```python
from build123d import *

# Parameters (mm, degrees)
BOSS_EXTRUDE1_DEPTH                            = 4
SKETCH3_R                                      = 2.15
BOSS_EXTRUDE2_DEPTH                            = 8
BOSS_EXTRUDE3_DEPTH                            = 8
CUT_EXTRUDE2_REACH                             = 34.144
SKETCH4_R                                      = 2.25
SKETCH4_4_W                                    = 12.7
SKETCH4_4_H                                    = 12.7
SKETCH4_4_R                                    = 2.25
CUT_EXTRUDE3_DEPTH                             = 8.5
BOSS_EXTRUDE4_DEPTH                            = 5.8
BOSS_EXTRUDE7_DEPTH                            = 3
CBORE_FOR_6_SOCKET_HEAD_CAP_SCREW1_D           = 3.6576
CBORE_FOR_6_SOCKET_HEAD_CAP_SCREW1_CBORE_D     = 7.14502
CBORE_FOR_6_SOCKET_HEAD_CAP_SCREW1_CBORE_DEPTH = 3.5052
SKETCH12_R                                     = 1.75
BOSS_EXTRUDE8_DEPTH                            = 2
CHAMFER1_SIZE                                  = 5
FILLET1_R                                      = 1


with BuildPart() as part:
    # Sketch2 → Boss-Extrude1 (new body)
    with BuildSketch(Plane.XY):
        with BuildLine():
            Line((15.5, 0), (20, 4.5))
            Line((20, 4.5), (20, 27))
            Line((20, 27), (1, 27))
            ThreePointArc((1, 27), (0.292893219, 26.707106781), (0, 26))
            Line((0, 26), (0, 1))
            ThreePointArc((0, 1), (0.292893219, 0.292893219), (1, 0))
            Line((1, 0), (15.5, 0))
        make_face()
    extrude(amount=BOSS_EXTRUDE1_DEPTH)

    # Sketch3 → Boss-Extrude2 (add)
    with BuildSketch(Plane.XY):
        with Locations((4.5, 22.5)):
            Circle(SKETCH3_R)
        with Locations((4.5, 4.5)):
            Circle(SKETCH3_R)
    extrude(amount=-BOSS_EXTRUDE2_DEPTH)

    # Sketch3<3> → Boss-Extrude3 (add)
    with BuildSketch(Plane.XY):
        with BuildLine():
            Line((4.5, 15), (4.5, 12))
            ThreePointArc((4.5, 12), (8.782801805, 10.656915518), (11.531693039, 7.108695652))
            ThreePointArc((11.531693039, 7.108695652), (12.997768364, 5.216311724), (15.281929326, 4.5))
            Line((15.281929326, 4.5), (20, 4.5))
            Line((20, 4.5), (20, 27))
            Line((20, 27), (12, 27))
            Line((12, 27), (12, 22.5))
            ThreePointArc((12, 22.5), (9.803300859, 17.196699141), (4.5, 15))
        make_face()
    extrude(amount=-BOSS_EXTRUDE3_DEPTH)

    # Cut-Extrude2: up to this face of the body (flat: up to its plane)
    cut_extrude2_end = Plane(part.part.faces().sort_by_distance((20, 15.75, -2))[0])
    # Sketch4 → Cut-Extrude2 (cut, up to the picked face)
    with BuildSketch(Plane(origin=(4.5, 0, 0), x_dir=(0, 0, -1), z_dir=(1, 0, 0)), mode=Mode.PRIVATE) as cut_extrude2_sk1:
        with Locations((8, 13.5)):
            Circle(SKETCH4_R)
    cut_extrude2_tool1 = split(extrude(cut_extrude2_sk1.sketch, amount=CUT_EXTRUDE2_REACH, mode=Mode.PRIVATE), bisect_by=cut_extrude2_end, keep=Keep.BOTH, mode=Mode.PRIVATE)
    add(cut_extrude2_tool1.solids().sort_by(Axis((4.5, 13.5, -8), (1, 0, 0)))[0], mode=Mode.SUBTRACT)

    # Sketch4<4> → Cut-Extrude3 (cut)
    with BuildSketch(Plane(origin=(4.5, 0, 0), x_dir=(0, 0, -1), z_dir=(1, 0, 0))):
        with Locations((8, 13.5)):
            Rectangle(SKETCH4_4_W, SKETCH4_4_H)
        with Locations((8, 13.5)):
            Circle(SKETCH4_4_R, mode=Mode.SUBTRACT)
    extrude(amount=CUT_EXTRUDE3_DEPTH, mode=Mode.SUBTRACT)

    # Sketch5 → Boss-Extrude4 (add)
    with BuildSketch(Plane(origin=(20, 0, 0), x_dir=(0, 0, -1), z_dir=(1, 0, 0))):
        with BuildLine():
            Line((1.45, 4.5), (1.45, 9.745003329))
            ThreePointArc((1.45, 9.745003329), (1.467285217, 17.28498845), (8, 21.05))
            Line((8, 21.05), (8, 27))
            Line((8, 27), (-4, 27))
            Line((-4, 27), (-4, 4.5))
            Line((-4, 4.5), (0, 4.5))
            Line((0, 4.5), (1.45, 4.5))
        make_face()
    extrude(amount=BOSS_EXTRUDE4_DEPTH)

    # Sketch8 → Boss-Extrude7 (add)
    with BuildSketch(Plane(origin=(25.8, 0, 0), x_dir=(0, 0, -1), z_dir=(1, 0, 0))):
        with BuildLine():
            Line((1.45, 4.5), (1.45, 9.745003329))
            ThreePointArc((1.45, 9.745003329), (1.467285217, 17.28498845), (8, 21.05))
            Line((8, 21.05), (8, 27))
            Line((8, 27), (-4, 27))
            Line((-4, 27), (-4, 4.5))
            Line((-4, 4.5), (1.45, 4.5))
        make_face()
        with BuildLine():
            Line((8, 15.75), (8, 21.05))
            ThreePointArc((8, 21.05), (1.467285217, 17.28498845), (1.45, 9.745003329))
            Line((1.45, 9.745003329), (1.45, 4.5))
            Line((1.45, 4.5), (8, 4.5))
            Line((8, 4.5), (8, 11.25))
            ThreePointArc((8, 11.25), (5.75, 13.5), (8, 15.75))
        make_face()
    extrude(amount=BOSS_EXTRUDE7_DEPTH)

    # CBORE for #6 Socket Head Cap Screw1 (through all)
    with Locations(Plane.XY.offset(4)):
        with Locations((16.5, 21.75)):
            CounterBoreHole(CBORE_FOR_6_SOCKET_HEAD_CAP_SCREW1_D / 2, CBORE_FOR_6_SOCKET_HEAD_CAP_SCREW1_CBORE_D / 2, CBORE_FOR_6_SOCKET_HEAD_CAP_SCREW1_CBORE_DEPTH)

    # Sketch12 → Boss-Extrude8 (add)
    with BuildSketch(Plane(origin=(0, 0, -8), x_dir=(-1, 0, 0), z_dir=(0, 0, -1))):
        with Locations(Location((-16.5, 7.875, 0), (0, 0, 180))):
            Circle(SKETCH12_R)
    extrude(amount=BOSS_EXTRUDE8_DEPTH)

    # Chamfer1
    chamfer1_edges = [part.edges().sort_by_distance(p)[0] for p in [
        (28.8, 27, -2),
    ]]
    chamfer(chamfer1_edges, length=CHAMFER1_SIZE)

    # Fillet1
    fillet1_edges = [part.edges().sort_by_distance(p)[0] for p in [
        (28.8, 4.5, -2),
    ]]
    fillet(fillet1_edges, radius=FILLET1_R)


solid = part.part
```
Can you work these out from the model? Positions are in its coordinate system, mm. A direction names the side the tool comes from. Coordinates: 2 decimals unless noted, no trailing zeros. Order: outer loops, then holes, each group sorted by start corner. A loop starts at its lowest first (then second) coordinate and runs counter-clockwise, first axis right, second up. Notation, with made-up numbers: (30, 79) - (86, 79) arc R22 ccw to (86, 96) - close; hole circle Ø8 at (24, -8). An arc over 180 degrees is marked (long way). Answer in a Markdown table with one row per item.
1. If I drill on line 1 along Y through (x, z) = (16.5, 2); line 2 along X through (y, z) = (21.5, -1); line 3 along X through (y, z) = (10.5, -1.75), over which ranges is the centre line in solid material (lowest first)?
Reply:
| item | result |
|---|---|
| line 1 | y = 1 to 18.18, 25.32 to 27 |
| line 2 | x = 2.6 to 6.4, 11.93 to 14.69, 18.31 to 28.8 |
| line 3 | x = 13 to 20, 25.8 to 28.8 |
2. Suppose I cut it at D-D (x = 22.75). Please give me the cut outline in (y, z) (3 decimals).
Reply:
| item | result |
|---|---|
| outline | (4.5, -1.45) - (9.745, -1.45) arc R7.55 cw to (21.05, -8) - (27, -8) - (27, 4) - (4.5, 4) - close |
3. Suppose I cut it at A-A (x = 16.5). Please give me the cut outline in (y, z) (3 decimals), and give its area (3 significant figures).
Reply:
| item | result |
|---|---|
| outline | (1, 0) - (4.5, 0) - (4.5, -8) - (6.125, -8) - (6.125, -10) - (9.625, -10) - (9.625, -8) - (11.25, -8) arc R2.25 cw to (15.75, -8) - (19.921, -8) - (19.921, 0.495) - (18.177, 0.495) - (18.177, 4) - (1, 4) - close; (23.579, -8) - (27, -8) - (27, 4) - (25.323, 4) - (25.323, 0.495) - (23.579, 0.495) - close |
| area | 227 mm^2 |
4. If we mould it in two halves opening along Y, with no side actions, what happens to faces 5 (the flat face through (26.3, 24.5, -2.1)), 6 (the cylindrical face through (27.28, 13.45, -5.75)), 7 (the flat face through (8, 0, 2)), 8 (the flat face through (27, 8, -8))? For each: pulls with the +Y half, pulls with the -Y half, needs draft (parallel to the pull), parting line crosses it, or undercut.
Reply:
| item | result |
|---|---|
| face 5 | pulls with the +Y half |
| face 6 | undercut |
| face 7 | pulls with the -Y half |
| face 8 | needs draft |
5. For faces 1 (the cylindrical face through (2.35, 4.59, -3.94)), 2 (the cylindrical face through (12.97, 5.236, -3.944)), 3 (the flat face through (18, 20, 0.495)), 4 (the flat face through (12, 19.85, -5)), which set-ups out of +Z, -Z, +X, -X, +Y, -Y let a thin tool reach every point of the face, with its end or its side?
Reply:
| item | result |
|---|---|
| face 1 | -Z |
| face 2 | -Z, -Y |
| face 3 | +Z |
| face 4 | -Z, -X |
6. For pin 1 (3.5 mm diameter, centred on x = 3.5, y = 22, fed in from -Z); pin 2 (2 mm diameter, centred on x = 14.5, y = 7, fed in from -Z); pin 3 (1.6 mm diameter, centred on x = 12, z = -3.5, fed in from -Y); pin 4 (3.5 mm diameter, centred on y = 26, z = -3, fed in from -X), each with a flat end and sliding along its axis, tell me the tip position at first contact or that it passes through.
Reply:
| item | result |
|---|---|
| pin 1 | stops at z = -8 |
| pin 2 | stops at z = -10 |
| pin 3 | stops at y = 5.36 |
| pin 4 | stops at x = 3.25 |
7. Suppose I cut it at B-B (z = -6.25). Please give me the cut outline in (x, y), and give its area (3 significant figures).
Reply:
| item | result |
|---|---|
| outline | circle Ø4.3 at (4.5, 4.5); circle Ø4.3 at (4.5, 22.5); (11.52, 7.15) arc R7.5 cw to (11.53, 7.11) arc R4 ccw to (15.28, 4.5) - (20, 4.5) - (20, 12.09) - (13, 12.09) - (13, 7.15) - close; (11.52, 19.85) - (13, 19.85) - (13, 14.91) - (20, 14.91) - (20, 20.84) - (25.8, 20.84) - (25.8, 14.91) - (28.8, 14.91) - (28.8, 22) - (23.8, 27) - (12, 27) - (12, 22.5) arc R7.5 cw to start; (25.8, 4.5) - (27.8, 4.5) arc R1 ccw to (28.8, 5.5) - (28.8, 12.09) - (25.8, 12.09) - close; hole circle Ø3.66 at (16.5, 21.75) |
| area | 247 mm^2 |
8. Suppose I cut it at C-C (z = -4.75). Please give me the cut outline in (x, y), and give its area (3 significant figures).
Reply:
| item | result |
|---|---|
| outline | circle Ø4.3 at (4.5, 4.5); circle Ø4.3 at (4.5, 22.5); (11.52, 7.15) arc R7.5 cw to (11.53, 7.11) arc R4 ccw to (15.28, 4.5) - (20, 4.5) - (20, 20.31) - (25.8, 20.31) - (25.8, 4.5) - (27.8, 4.5) arc R1 ccw to (28.8, 5.5) - (28.8, 22) - (23.8, 27) - (12, 27) - (12, 22.5) arc R7.5 cw to (11.52, 19.85) - (13, 19.85) - (13, 7.15) - close; hole circle Ø3.66 at (16.5, 21.75) |
| area | 278 mm^2 |
